The drawing under review shows one solid part. Ordinate dimensions are in mm from its lowest x, y, z. Coordinates: 2 decimals unless noted, no trailing zeros. Loops run counter-clockwise (first coordinate to the right, second up) from the corner with the lowest first, then second, coordinate; pieces in that order, holes last. Notation, with made-up numbers: M -22,61.5 L 2,61.5 A6 cw 2,70.5 Z; hole C -27.5,84.5 d11. An arc over 180 degrees is marked long. Answer as a JSON object with one key per item and string values. Group by question number.
1. Consider section D-D (x = 48.5). State the section outline as (y, z) points.
2. Consider section A-A (y = 50). State the section outline as (x, z) points.
3. Insertion check: pin 1 (12 mm diameter, centred on x = 45, y = 50, fed in from -Z); pin 2 (4.5 mm diameter, centred on x = 98, y = 90, fed in from +Z); pin 3 (1.3 mm diameter, centred on y = 35.5, z = 1.5, fed in from +X). Each pin has a flat end and moves straight along its axis. Give the tip position at first contact, or say it passes through.
4. Consider section B-B (z = 3.55). Count the separate pieces of the cut face and the enclosed holes in it, then the cut area to 3 significant figures.
5. Consider section C-C (x = 79.5). State the section outline as (y, z) points, then the cut area to 3 significant figures.
6. To check wall thickness, follow probe 1 along Y at (x, z) = (70, 0.9); probe 2 along Y at (x, z) = (42, 0.35); probe 3 along X at (y, z) = (11, 0.55). State the ranges of each line that lie inside material, in increasing order.
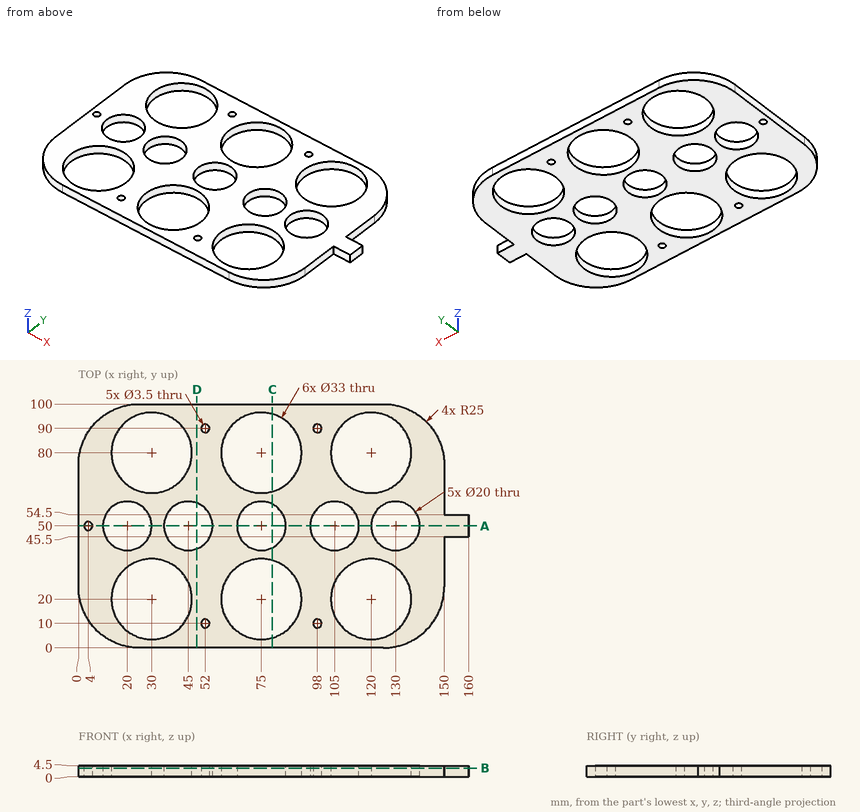
Findings below:
{
 "1": {"outline": "M 0,0 L 40.63,0 L 40.63,4.5 L 0,4.5 Z; M 59.37,0 L 100,0 L 100,4.5 L 59.37,4.5 Z"},
 "2": {"outline": "M 0,0 L 2.25,0 L 2.25,4.5 L 0,4.5 Z; M 5.75,0 L 10,0 L 10,4.5 L 5.75,4.5 Z; M 30,0 L 35,0 L 35,4.5 L 30,4.5 Z; M 55,0 L 65,0 L 65,4.5 L 55,4.5 Z; M 85,0 L 95,0 L 95,4.5 L 85,4.5 Z; M 115,0 L 120,0 L 120,4.5 L 115,4.5 Z; M 140,0 L 160,0 L 160,4.5 L 140,4.5 Z"},
 "3": {"pin 1": "passes through", "pin 2": "stops at z = 4.5", "pin 3": "stops at x = 150"},
 "4": {"separate pieces": "1", "enclosed holes": "16", "area": "7,800 mm^2"},
 "5": {"outline": "M 0,0 L 4.13,0 L 4.13,4.5 L 0,4.5 Z; M 35.87,0 L 41.07,0 L 41.07,4.5 L 35.87,4.5 Z; M 58.93,0 L 64.13,0 L 64.13,4.5 L 58.93,4.5 Z; M 95.87,0 L 100,0 L 100,4.5 L 95.87,4.5 Z", "area": "83.9 mm^2"},
 "6": {"probe 1": "y = 0 to 4.28, 35.72 to 41.34, 58.66 to 64.28, 95.72 to 100", "probe 2": "y = 0 to 8.68, 31.32 to 40.46, 59.54 to 68.68, 91.32 to 100", "probe 3": "x = 4.29 to 16.17, 43.83 to 50.56, 53.44 to 61.17, 88.83 to 96.56, 99.44 to 106.17, 133.83 to 145.71"}
}
